Autodesk Inventor part; units mm, degrees
ref_plane "YZ Plane" through (0, 0, 0) normal (1, 0, 0) x (0, 1, 0)
ref_plane "XZ Plane" through (0, 0, 0) normal (0, 1, 0) x (-1, 0, 0)
ref_plane "XY Plane" through (0, 0, 0) normal (0, 0, 1) x (1, 0, 0)
sketch "Sketch1" plane through (0, 0, 0) normal (0, 0, 1) x (1, 0, 0)
  line L0 (-15, 7.5) -> (15, 7.5)
  line L1 (15, 7.5) -> (15, -7.5)
  line L2 (15, -7.5) -> (-15, -7.5)
  line L3 (-15, -7.5) -> (-15, 7.5)
  line L4 (-15, 7.5) -> (15, -7.5) construction
  line L5 (15, 7.5) -> (-15, -7.5) construction
  line L6 (-15, 0) -> (-7, 0) construction
  line L7 (-7, 0) -> (-7, -2.5) construction
  line L8 (0, 7.5) -> (0, -7.5) construction
  circle A0 centre (-7, -2.5) radius 1.6
  line L9 (0, -7.5) -> (0, 7.5) construction
  circle A1 centre (-7, 2.5) radius 1.6
  circle A2 centre (7, -2.5) radius 1.6
  circle A3 centre (7, 2.5) radius 1.6
  line L10 (7, 2.5) -> (-7, 2.5) construction
  point P0 (0, 0)
  dimension "d0" = 30
  dimension "d1" = 15
  dimension "d3" = 2.5
  dimension "d4" = 3.2
  dimension "d11" = 14
extrude "Extrusion1" add sketch "Sketch1" along normal blind 30
sketch "Sketch2" plane through (-15, -7.5, 0) normal (0, -1, 0) x (1, 0, 0)
  line L0 (0, 30) -> (30, 30)
  line L1 (0, 30) -> (30, 30)
  line L2 (30, 30) -> (30, 15)
  line L3 (30, 15) -> (0, 15)
  line L4 (0, 15) -> (0, 30)
  point P0 (15, 0)
  dimension "d7" = 30
  dimension "d8" = 15
extrude "Extrusion2" add sketch "Sketch2" along normal blind 50
sketch "Sketch3" plane through (-15, -57.5, 0) normal (0, -1, 0) x (1, 0, 0)
  line L0 (0, 15) -> (30, 15)
  line L1 (15, 15) -> (15, 22.5) construction
  line L2 (15, 22.5) -> (3.85, 22.5) construction
  line L3 (15, 22.5) -> (26.15, 22.5) construction
  line L4 (3.85, 28.45) -> (26.15, 28.45)
  line L5 (26.15, 28.45) -> (26.15, 16.55)
  line L6 (26.15, 16.55) -> (3.85, 16.55)
  line L7 (3.85, 16.55) -> (3.85, 28.45)
  line L8 (3.85, 28.45) -> (26.15, 16.55) construction
  line L9 (26.15, 28.45) -> (3.85, 16.55) construction
  line L10 (0, 30) -> (30, 30)
  line L11 (30, 30) -> (30, 15)
  line L12 (30, 15) -> (0, 15)
  line L13 (0, 15) -> (0, 30)
  line L14 (0, 30) -> (30, 15) construction
  line L15 (30, 30) -> (0, 15) construction
  point P0 (15, 0)
  dimension "d12" = 7.5
  dimension "d14" = 11.15
  dimension "d15" = 11.15
  dimension "d19" = 22.3
  dimension "d20" = 11.9
  dimension "d21" = 15
extrude "Extrusion3" add sketch "Sketch3" along normal blind 15
sketch "Sketch4" plane through (-15, -72.5, 0) normal (0, -1, 0) x (1, 0, 0)
  line L0 (30, 30) -> (0, 30)
  line L1 (0, 30) -> (3.85, 30)
  line L2 (3.85, 30) -> (3.85, 15)
  line L3 (3.85, 15) -> (0, 15)
  line L4 (0, 15) -> (0, 30)
  line L5 (30, 0) -> (30, 30)
  line L6 (30, 30) -> (26.15, 30)
  line L7 (26.15, 30) -> (26.15, 15)
  line L8 (26.15, 15) -> (30, 15)
  line L9 (30, 15) -> (30, 30)
  point P0 (15, 0)
  dimension "d24" = 15
  dimension "d25" = 15
extrude "Extrusion4" cut sketch "Sketch4" against normal blind 12
sketch "Sketch5" plane through (-11.15, -72.5, 15) normal (-1, 0, 0) x (0, 0, 1)
  line L0 (13.45, 0) -> (15, 0)
  line L1 (15, 0) -> (0, 0)
  line L2 (0, 0) -> (0, 4)
  line L3 (0, 4) -> (15, 4)
  line L4 (15, 4) -> (15, 0)
  point P0 (-15, 72.5)
  point P1 (13.45, 0)
  dimension "d28" = 15
  dimension "d29" = 4
extrude "Extrusion5" add sketch "Sketch5" along normal blind 5
sketch "Sketch6" plane through (-15, -72.5, 0) normal (0, -1, 0) x (1, 0, 0)
  line L0 (3.85, 28.45) -> (3.85, 16.55)
  circle A0 centre (1.5, 22.5) radius 1.6
  line L1 (26.15, 28.45) -> (3.85, 28.45) construction
  line L2 (15, 28.45) -> (15, 16.55) construction
  line L3 (3.85, 16.55) -> (26.15, 16.55) construction
  point P0 (15, 0)
  dimension "d33" = 3.2
  dimension "d56" = 13.5
extrude "Extrusion6" cut sketch "Sketch6" against normal blind 4
mirror "Mirror1" about plane through (0, 0, 0) normal (1, 0, 0) of "Extrusion5"
mirror "Mirror2" about plane through (0, 0, 0) normal (1, 0, 0) of "Extrusion6"
fillet "Fillet1" radius 2 13 edges at (15, -7.5, 7.5) (15, 7.5, 15) (-15, -7.5, 7.5) (-15, 7.5, 15) (-15, -34, 15) (15, -34, 15) (-15, -26.5, 30) (15, -26.5, 30) (0, 7.5, 30) (16.15, -70.5, 15) (-16.15, -70.5, 15) (-16.15, -70.5, 30) (16.15, -70.5, 30)
properties part number "attachment of brush"
Check sheet for the modelled part. Datum: model origin and axes. Units: mm. A direction names the side the tool comes from. Give positions to 0.01 mm unless a question says otherwise; leave off trailing zeros. Write each loop counter-clockwise with the first axis right and the second up, starting at its lowest first coordinate (ties: lowest second). Pieces come first, ordered by that corner, then holes. Notation, with made-up numbers: (77.5, 43) -> (125.5, 43) arc R9 ccw to (125.5, 60) -> close; hole circle Ø11 at (12, -3.5). An arc over 180 degrees is marked (long way). One line per item, written item: value. Start each with the question number.
Item 1: Draft check along X on faces 4 (the cylindrical face through (14.4, -33.39, 15.57)), 5 (the flat face through (0, -7.5, 7)), 6 (the flat face through (0, -57.5, 23)). Enter one of: +X half, -X half, draft (parallel to the pull), parting line (faces both ways), or undercut.
Item 2: Section check A-A on z = 22.5. State how many separate pieces and enclosed holes the cut face has, then the cut area to 3 significant figures.
Item 3: Section check C-C on y = 2.5. Record the cut outline in (x, z).
Item 4: Section check B-B on z = 26. Record the cut outline in (x, y), then the cut area to 3 significant figures.
Item 5: Material ranges on probe 1 along Y at (x, z) = (-7, 10); probe 2 along Y at (x, z) = (7, 20); probe 3 along Z at (x, y) = (6, -67), recorded low to high. Write a range as from..to.
Item 6: Section check D-D on x = -7. Record the cut outline in (y, z).
Item 7: Tool access check on faces 1 (the flat face through (-11.15, -70, 22)), 2 (the cylindrical face through (-14.43, -27.04, 29.4)), 3 (the flat face through (11.15, -65, 29)). Record the directions out of +Z, -Z, +X, -X, +Y, -Y that give a thin tool (end or side, any length) a straight path to the whole face; none if there is none.
Item 8: Gauge pin test, flat ends, axial feed: pin 1 (1.5 mm diameter, centred on x = -15, z = 21.5, fed in from +Y); pin 2 (4.5 mm diameter, centred on x = -5.5, z = 4, fed in from -Y); pin 3 (1.5 mm diameter, centred on x = -7.5, y = -26.5, fed in from -Z); pin 4 (3 mm diameter, centred on x = 7, y = 2.5, fed in from +Z). Record the tip position at first contact, or that the pin passes through.
Results list:
1. face 4: +X half
1. face 5: draft
1. face 6: undercut
2. separate pieces: 5
2. enclosed holes: 4
2. area: 1,950 mm²
3. outline: (-15, 0) -> (-8.6, 0) -> (-8.6, 30) -> (-13, 30) arc R2 ccw to (-15, 28) -> close; (-5.4, 0) -> (5.4, 0) -> (5.4, 30) -> (-5.4, 30) -> close; (8.6, 0) -> (15, 0) -> (15, 28) arc R2 ccw to (13, 30) -> (8.6, 30) -> close
4. outline: (-16.15, -72.5) -> (-11.15, -72.5) -> (-11.15, -68.5) -> (-16.15, -68.5) -> close; (-15, -60.5) -> (-11.15, -60.5) -> (-11.15, -57.5) -> (11.15, -57.5) -> (11.15, -60.5) -> (15, -60.5) -> (15, 5.5) arc R2 ccw to (13, 7.5) -> (-13, 7.5) arc R2 ccw to (-15, 5.5) -> close; (11.15, -72.5) -> (16.15, -72.5) -> (16.15, -68.5) -> (11.15, -68.5) -> close; hole circle Ø3.2 at (-7, -2.5); hole circle Ø3.2 at (-7, 2.5); hole circle Ø3.2 at (7, -2.5); hole circle Ø3.2 at (7, 2.5)
4. area: 1,980 mm²
5. probe 1: -7.5..-4.1, -0.9..0.9, 4.1..7.5
5. probe 2: -57.5..-4.1, -0.9..0.9, 4.1..7.5
5. probe 3: 15..16.55, 28.45..30
6. outline: (-72.5, 15) -> (-7.5, 15) -> (-7.5, 0) -> (-4.1, 0) -> (-4.1, 30) -> (-72.5, 30) -> (-72.5, 28.45) -> (-57.5, 28.45) -> (-57.5, 16.55) -> (-72.5, 16.55) -> close; (-0.9, 0) -> (0.9, 0) -> (0.9, 30) -> (-0.9, 30) -> close; (4.1, 0) -> (7.5, 0) -> (7.5, 28) arc R2 ccw to (5.5, 30) -> (4.1, 30) -> close
7. face 1: -Y
7. face 2: +Z, -X, +Y
7. face 3: +Z, -Z, +X
8. pin 1: y = 7.06
8. pin 2: y = -7.5
8. pin 3: z = 15
8. pin 4: through
